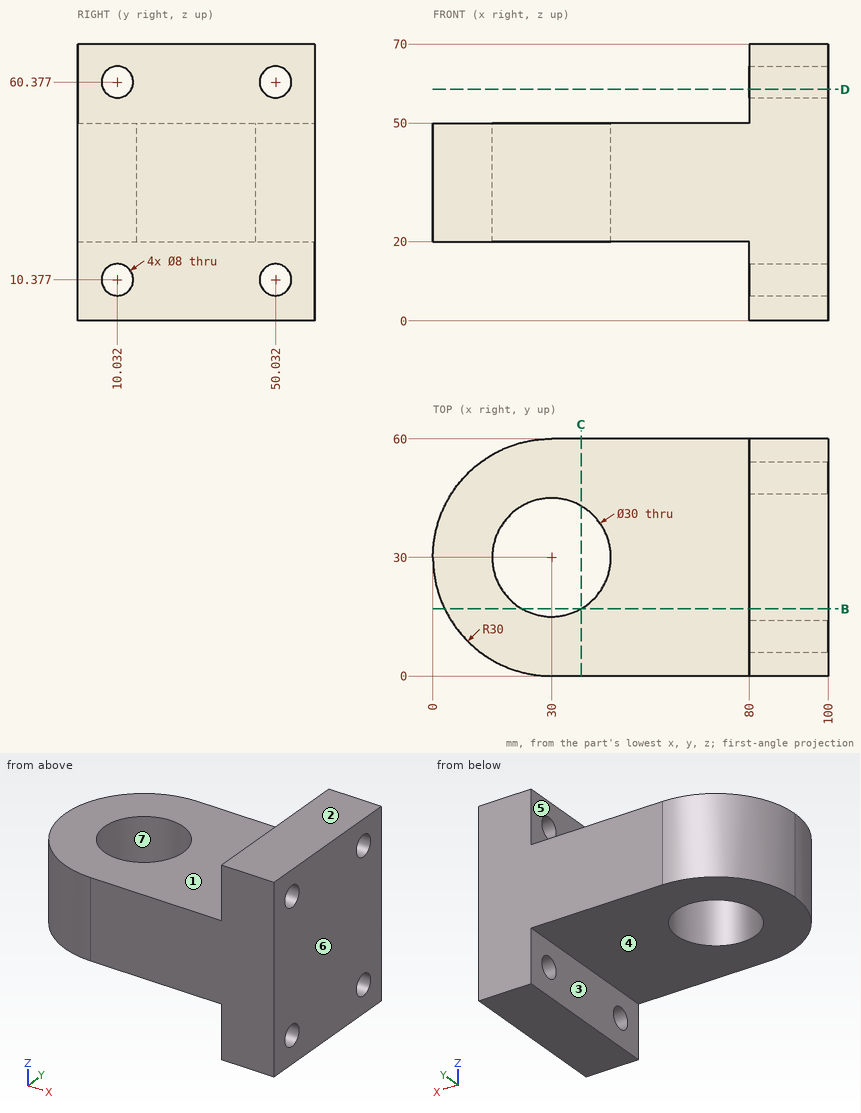
Geometry check sheet. Reference: drawing and pictorial views, mm from the part's lowest x, y, z. A direction names the side the tool comes from. Give positions to 0.01 mm unless a question says otherwise; leave off trailing zeros. Loops run counter-clockwise (first coordinate to the right, second up) from the corner with the lowest first, then second, coordinate; pieces in that order, holes last.
1. Mould release check, pull along X, two halves, no side actions. Record for the marked faces 4, 5, 6 and 7: released by +X, released by -X, zero draft, split by the parting line, or undercut.
2. Go/stop test with flat-tipped pins: pin 1 Ø9 at (y, z) = (50.03, 60.38) entering from -X; pin 2 Ø10 at (y, z) = (19, 50.5) entering from -X; pin 3 Ø5 at (y, z) = (45.5, 26.5) entering from -X. Record where each tip stops, or that it passes through.
3. Section check C-C, the plane x = 37.5. Enter the section's corners in (y, z).
4. Section check B-B, the plane y = 17. Enter the section's corners in (x, z), then the cut area to 3 significant figures.
5. Thickness scan on line 1 (X direction, y = 46.5, z = 19); line 2 (Z direction, x = 43.5, y = 9); line 3 (X direction, y = 22, z = 31) (1 decimal). Record the ranges inside material, lowest first.
6. Section check D-D, the plane z = 58.5. Enter the section's corners in (x, y) (1 decimal).
7. Set-up check for the marked faces 1, 2 and 3: record each of +Z, -Z, +X, -X, +Y, -Y from which the full face is reachable in a straight line by a thin tool's end or side.
Geometry says:
1. face 4: zero draft
1. face 5: released by -X
1. face 6: released by +X
1. face 7: undercut
2. pin 1: stops at x = 80
2. pin 2: stops at x = 0.61
2. pin 3: stops at x = 2.96
3. outline: (0, 20) - (17.01, 20) - (17.01, 50) - (0, 50) - close; (42.99, 20) - (60, 20) - (60, 50) - (42.99, 50) - close
4. outline: (2.96, 20) - (22.52, 20) - (22.52, 50) - (2.96, 50) - close; (37.48, 20) - (80, 20) - (80, 0) - (100, 0) - (100, 70) - (80, 70) - (80, 50) - (37.48, 50) - close
4. area: 3,260 mm2
5. line 1: x = 80 to 100
5. line 2: z = 20 to 50
5. line 3: x = 1.1 to 17.3, 42.7 to 100
6. outline: (80, 0) - (100, 0) - (100, 6.5) - (80, 6.5) - close; (80, 13.6) - (100, 13.6) - (100, 46.5) - (80, 46.5) - close; (80, 53.6) - (100, 53.6) - (100, 60) - (80, 60) - close
7. face 1: +Z, -X, +Y, -Y
7. face 2: +Z, +X, -X, +Y, -Y
7. face 3: -Z, -X, +Y, -Y
